from build123d import *

# Parameters (mm, degrees)
SKETCH1_W                                = 53
SKETCH1_H                                = 53
SKETCH1_W_2                              = 41
SKETCH1_H_2                              = 41
BOSS_EXTRUDE1_DEPTH                      = 40
SKETCH2_W                                = 53
SKETCH2_H                                = 53
BOSS_EXTRUDE2_DEPTH                      = 6
SKETCH3_W                                = 53
SKETCH3_H                                = 80
SKETCH3_W_2                              = 41
SKETCH3_H_2                              = 68
BOSS_EXTRUDE3_DEPTH                      = 31
BOSS_EXTRUDE4_DEPTH                      = 31
BOSS_EXTRUDE5_START                      = -6
BOSS_EXTRUDE5_DEPTH                      = 6
SKETCH6_W                                = 41
SKETCH6_H                                = 12
CUT_EXTRUDE1_DEPTH                       = 25
CBORE_FOR_M3_SHCS2_D                     = 3.4
CBORE_FOR_M3_SHCS2_CBORE_D               = 6.5
CBORE_FOR_M3_SHCS2_CBORE_DEPTH           = 3
CUT_EXTRUDE2_REACH                       = 166.954
SKETCH14_W                               = 41
SKETCH14_H                               = 41
CUT_EXTRUDE3_DEPTH                       = 40
CUT_EXTRUDE4_REACH                       = 127.3
SKETCH15_W                               = 19.88190451
SKETCH15_H                               = 41
CBORE_FOR_M5_SHCS1_D                     = 5.5
CBORE_FOR_M5_SHCS1_DEPTH                 = 6
CBORE_FOR_M5_SHCS1_CBORE_D               = 10
CBORE_FOR_M5_SHCS1_CBORE_DEPTH           = 5
CBORE_FOR_M5_SHCS1_ON_FACE_2_D           = 5.5
CBORE_FOR_M5_SHCS1_ON_FACE_2_DEPTH       = 6
CBORE_FOR_M5_SHCS1_ON_FACE_2_CBORE_D     = 10
CBORE_FOR_M5_SHCS1_ON_FACE_2_CBORE_DEPTH = 5
CBORE_FOR_M5_SHCS1_ON_FACE_3_D           = 5.5
CBORE_FOR_M5_SHCS1_ON_FACE_3_DEPTH       = 6
CBORE_FOR_M5_SHCS1_ON_FACE_3_CBORE_D     = 10
CBORE_FOR_M5_SHCS1_ON_FACE_3_CBORE_DEPTH = 5
CUT_EXTRUDE5_START                       = -26.5
CUT_EXTRUDE5_DEPTH                       = 53


with BuildPart() as part:
    # Sketch1 → Boss-Extrude1 (new body)
    with BuildSketch(Plane(origin=(0, 0, 0), x_dir=(1, 0, 0), z_dir=(0, 1, 0))):
        Rectangle(SKETCH1_W, SKETCH1_H)
        Rectangle(SKETCH1_W_2, SKETCH1_H_2, mode=Mode.SUBTRACT)
    extrude(amount=BOSS_EXTRUDE1_DEPTH)

    # Sketch2 → Boss-Extrude2 (add)
    with BuildSketch(Plane(origin=(0, 40, 0), x_dir=(1, 0, 0), z_dir=(0, 1, 0))):
        Rectangle(SKETCH2_W, SKETCH2_H)
    extrude(amount=BOSS_EXTRUDE2_DEPTH)

    # Sketch3 → Boss-Extrude3 (add)
    with BuildSketch(Plane(origin=(13.2248366, -3.543584287, 0), x_dir=(0, 0, -1), z_dir=(-0.9659258262890681, 0.25881904510252135, 0))):
        with Locations((0, -71.291292705)):
            Rectangle(SKETCH3_W, SKETCH3_H)
        with Locations((0, -71.291292705)):
            Rectangle(SKETCH3_W_2, SKETCH3_H_2, mode=Mode.SUBTRACT)
    extrude(amount=BOSS_EXTRUDE3_DEPTH)

    # Sketch4 → Boss-Extrude4 (add)
    with BuildSketch(Plane(origin=(13.2248366, -3.543584287, 0), x_dir=(0, 0, -1), z_dir=(0.9659258262890681, -0.25881904510252135, 0))):
        with BuildLine():
            Line((-32.3, 148.691292705), (32.3, 148.691292705))
            ThreePointArc((32.3, 148.691292705), (51, 129.991292705), (32.3, 111.291292705))
            Line((32.3, 111.291292705), (-32.3, 111.291292705))
            ThreePointArc((-32.3, 111.291292705), (-51, 129.991292705), (-32.3, 148.691292705))
        make_face()
        with BuildLine():
            Line((-32.3, 142.691292705), (32.3, 142.691292705))
            ThreePointArc((32.3, 142.691292705), (45, 129.991292705), (32.3, 117.291292705))
            Line((32.3, 117.291292705), (-32.3, 117.291292705))
            ThreePointArc((-32.3, 117.291292705), (-45, 129.991292705), (-32.3, 142.691292705))
        make_face(mode=Mode.SUBTRACT)
    extrude(amount=-BOSS_EXTRUDE4_DEPTH)

    # Sketch5 → Boss-Extrude5 (add)
    with BuildSketch(Plane(origin=(-16.718864015, 4.479806111, 0), x_dir=(0, 0, 1), z_dir=(-0.9659258262890681, 0.25881904510252135, 0)).offset(BOSS_EXTRUDE5_START)):
        with BuildLine():
            Line((-20.5, 42.984867739), (20.5, 42.984867739))
            Line((20.5, 42.984867739), (26.5, 42.984867739))
            Line((26.5, 42.984867739), (26.5, 111.291292705))
            Line((26.5, 111.291292705), (32.3, 111.291292705))
            ThreePointArc((32.3, 111.291292705), (51, 129.991292705), (32.3, 148.691292705))
            Line((32.3, 148.691292705), (-32.3, 148.691292705))
            ThreePointArc((-32.3, 148.691292705), (-51, 129.991292705), (-32.3, 111.291292705))
            Line((-32.3, 111.291292705), (-26.5, 111.291292705))
            Line((-26.5, 111.291292705), (-26.5, 42.984867739))
            Line((-26.5, 42.984867739), (-20.5, 42.984867739))
        make_face()
    extrude(amount=BOSS_EXTRUDE5_DEPTH)

    # Sketch6 → Cut-Extrude1 (cut)
    with BuildSketch(Plane(origin=(13.2248366, -3.543584287, 0), x_dir=(0, 0, -1), z_dir=(0.9659258262890681, -0.25881904510252135, 0))):
        with Locations((0, 111.291292705)):
            Rectangle(SKETCH6_W, SKETCH6_H)
    extrude(amount=-CUT_EXTRUDE1_DEPTH, mode=Mode.SUBTRACT)

    # CBORE for M3 SHCS2 (through all)
    with Locations(Plane(origin=(-16.718864015, 4.479806111, 0), x_dir=(0, 0, 1), z_dir=(-0.9659258262890681, 0.25881904510252135, 0))):
        with Locations((22.5, 129.991292705), (-22.5, 129.991292705)):
            CounterBoreHole(CBORE_FOR_M3_SHCS2_D / 2, CBORE_FOR_M3_SHCS2_CBORE_D / 2, CBORE_FOR_M3_SHCS2_CBORE_DEPTH)

    # Sketch13 → Cut-Extrude2 (cut, up to next)
    with BuildSketch(Plane.XY, mode=Mode.PRIVATE) as cut_extrude2_sk1:
        Polygon((49.457249301, 131.677620792), (44.280868399, 112.359104266), (20.132722741, 118.829580394), (25.309103643, 138.148096919), align=None)
    cut_extrude2_tool1 = extrude(cut_extrude2_sk1.sketch, amount=CUT_EXTRUDE2_REACH, mode=Mode.PRIVATE) & part.part
    add(cut_extrude2_tool1.solids().sort_by_distance((34.794986, 125.253601, 0))[0], mode=Mode.SUBTRACT)

    # Sketch14 → Cut-Extrude3 (cut)
    with BuildSketch(Plane.XZ):
        Rectangle(SKETCH14_W, SKETCH14_H)
    extrude(amount=-CUT_EXTRUDE3_DEPTH, mode=Mode.SUBTRACT)

    # Sketch15 → Cut-Extrude4 (cut, up to next)
    with BuildSketch(Plane(origin=(0, 46, 0), x_dir=(1, 0, 0), z_dir=(0, 1, 0)), mode=Mode.PRIVATE) as cut_extrude4_sk1:
        with Locations((10.559047745, 0)):
            Rectangle(SKETCH15_W, SKETCH15_H)
    cut_extrude4_tool1 = extrude(cut_extrude4_sk1.sketch, amount=-CUT_EXTRUDE4_REACH, mode=Mode.PRIVATE) & part.part
    add(cut_extrude4_tool1.solids().sort_by_distance((10.559048, 46, 0))[0], mode=Mode.SUBTRACT)

    # CBORE for M5 SHCS1
    with Locations(Plane(origin=(0, 23, -26.5), x_dir=(-1, 0, 0), z_dir=(0, 0, -1))):
        with Locations((0, 0)):
            CounterBoreHole(CBORE_FOR_M5_SHCS1_D / 2, CBORE_FOR_M5_SHCS1_CBORE_D / 2, CBORE_FOR_M5_SHCS1_CBORE_DEPTH, depth=CBORE_FOR_M5_SHCS1_DEPTH)

    # CBORE for M5 SHCS1 on face 2
    with Locations(Plane(origin=(-26.5, 23, 0), x_dir=(0, 0, -1), z_dir=(-1, 0, 0))):
        with Locations((0, 0)):
            CounterBoreHole(CBORE_FOR_M5_SHCS1_ON_FACE_2_D / 2, CBORE_FOR_M5_SHCS1_ON_FACE_2_CBORE_D / 2, CBORE_FOR_M5_SHCS1_ON_FACE_2_CBORE_DEPTH, depth=CBORE_FOR_M5_SHCS1_ON_FACE_2_DEPTH)

    # CBORE for M5 SHCS1 on face 3
    with Locations(Plane(origin=(0, 23, 26.5), x_dir=(1, 0, 0), z_dir=(0, 0, 1))):
        with Locations((0, 0)):
            CounterBoreHole(CBORE_FOR_M5_SHCS1_ON_FACE_3_D / 2, CBORE_FOR_M5_SHCS1_ON_FACE_3_CBORE_D / 2, CBORE_FOR_M5_SHCS1_ON_FACE_3_CBORE_DEPTH, depth=CBORE_FOR_M5_SHCS1_ON_FACE_3_DEPTH)

    # Cut-Extrude5: read off the stored shape, not the designer's step
    # Cut-Extrude5 outline → Cut-Extrude5 (cut)
    with BuildSketch(Plane.XY.offset(CUT_EXTRUDE5_START)):
        Polygon((14.174337148, 0), (26.5, 0), (26.5, 46), align=None)
    extrude(amount=CUT_EXTRUDE5_DEPTH, mode=Mode.SUBTRACT)


solid = part.part
Model file for the job. Use its own axes, mm. A direction names the side the tool comes from. Give positions to 0.01 mm unless a question says otherwise; leave off trailing zeros. Order: outer loops, then holes, each group sorted by start corner. A loop starts at its lowest first (then second) coordinate and runs counter-clockwise, first axis right, second up. Notation, with made-up numbers: (-16.75, 34) - (4.25, 34) arc R22 ccw to (4.25, 67) - close; hole circle Ø2 at (70.5, -36). An arc over 180 degrees is marked (long way). Write item = value, one per line. Start each with the question number.
1. Cut at A-A, the plane z = 0. List the corners of the cut face in (x, y).
2. Which spindle directions (+Z, -Z, +X, -X, +Y, -Y) get a long thin tool onto all of the face, cutting with end or side? Do faces 1 (the flat face through (23, 46, 0)), 2 (the cylindrical face through (35, 125, -45)), 3 (the flat face through (27.27, 107.91, 29.36)), 4 (the flat face through (32.38, 115.55, 44.06)). Say none if no direction does.
3. Drop flat-ended pins along their axis: P1, Ø13, axis at y = 23, z = 0, coming from the -X side; P2, Ø6.5, axis at y = 42, z = -2.5, coming from the +X side; P3, Ø6.5, axis at y = 23, z = 0, coming from the -X side; P4, Ø10, axis at x = 26, y = 62, coming from the +Z side. Give the stop position or say it passes through.
4. Cut at C-C, the plane x = 7. List the corners of the cut face in (y, z).
5. Two-plate mould, pull along Z, no slides. Class faces 5 (the cylindrical face through (-20.993, 20.273, -0.358)), 6 (the flat face through (37.21, 134.96, 44.06)), 7 (the flat face through (2.2, 20.8, 21.5)): pulls with the +Z half, pulls with the -Z half, needs draft (parallel to the pull), parting line crosses it, or undercut.
6. Cut at D-D, the plane y = 67.5. List the corners of the cut face in (x, z).
7. Cut at B-B, the plane z = -11.5. List the corners of the cut face in (x, y).
8. Probe line 1 along X through (y, z) = (33.5, -14); line 2 along Z through (x, y) = (-21, 23); line 3 along Z through (x, y) = (3.5, 10). List the from-to ranges inside material, lowest first.
Taken from the geometry:
q1.outline = (-26.5, 0) - (-20.5, 0) - (-20.5, 20.25) - (-21.5, 20.25) - (-21.5, 18) - (-26.5, 18) - close; (-26.5, 28) - (-21.5, 28) - (-21.5, 25.75) - (-20.5, 25.75) - (-20.5, 40) - (0.62, 40) - (0.62, 46) - (26.01, 140.76) - (50.16, 134.29) - (51.71, 140.08) - (21.77, 148.1) - (-5.59, 46) - (-26.5, 46) - close; (20.5, 23.61) - (26.5, 46) - (20.5, 46) - close
q2.face_1 = +X
q2.face_2 = none
q2.face_3 = +Z, -X, -Y
q2.face_4 = +Z, +X
q3.P1 = -26.5
q3.P2 = 26.3
q3.P3 = -21.5
q3.P4 = 26.5
q4.outline = (0, -26.5) - (93, -26.5) - (93, 26.5) - (0, 26.5) - (0, 20.5) - (69.82, 20.5) - (69.82, -20.5) - (0, -20.5) - close
q5.face_5 = undercut
q5.face_6 = needs draft
q5.face_7 = pulls with the +Z half
q6.outline = (0.17, -26.5) - (32.26, -26.5) - (32.26, -20.5) - (6.38, -20.5) - (6.38, 20.5) - (32.26, 20.5) - (32.26, 26.5) - (0.17, 26.5) - close
q7.outline = (-26.5, 0) - (-20.5, 0) - (-20.5, 40) - (0.62, 40) - (0.62, 46) - (26.01, 140.76) - (50.16, 134.29) - (51.71, 140.08) - (21.77, 148.1) - (-5.59, 46) - (-26.5, 46) - close; (20.5, 23.61) - (26.5, 46) - (20.5, 46) - close
q8.line_1 = -26.5 to -20.5, 20.5 to 23.15
q8.line_2 = -26.5 to -2.75, 2.75 to 26.5
q8.line_3 = -26.5 to -20.5, 20.5 to 26.5
